Geometry: final body of the model. Coordinates: model frame, mm. A direction names the side the tool comes from. Give positions to 0.01 mm unless a question says otherwise; leave off trailing zeros. Order: outer loops, then holes, each group sorted by start corner. A loop starts at its lowest first (then second) coordinate and runs counter-clockwise, first axis right, second up. Notation, with made-up numbers: (-40, 50.25) - (-25, 50.25) arc R7 cw to (-25, 54.25) - close; hole circle Ø11 at (40, -31.5). An arc over 180 degrees is marked (long way). Put each result on its own line as item: value. Start each with the question number.
1. Section A-A on y = 11.5. Return the cut outline in (x, z).
2. Ray query, line 1 along X through (y, z) = (3, 10.75); line 2 along Y through (x, z) = (27.5, 8.25); line 3 along Y through (x, z) = (-3.5, 4.5). Return the intervals inside material, ascending. Write a range as from..to.
3. Mould query, pull axis X, two halves, no side actions, for faces 1 (the flat face through (-31, 12.55, 6)), 2 (the flat face through (26, -1.25, 6)), 3 (the flat face through (-34.25, 7, 6)), 4 (the cylindrical face through (-29.626, 12.906, 6.084)). Classes: pulls with the +X half, pulls with the -X half, needs draft (parallel to the pull), parting line crosses it, or undercut.
4. Section C-C on x = 14. Return the cut outline in (y, z), plus the area to 3 significant figures.
5. First-contact query: P1, Ø3.5, axis at x = -26, z = 5.5, coming from the -Y side; P2, Ø2, axis at x = 23, z = 3.5, coming from the -Y side; P3, Ø1.9, axis at y = -3.5, z = 7, coming from the -X side. Flat tips, straight axial feed; report the tip coordinate or a pass-through.
6. Section D-D on y = -4.5. Return the cut outline in (x, z), plus the area to 3 significant figures.
7. Set-up query: faces 5 (the cylindrical face through (-29.606, 14.674, 6.084)), 6 (the flat face through (31.75, 7, 6)), 7 (the flat face through (-6.25, -4, 6)). Return all of +Z, -Z, +X, -X, +Y, -Y with unobstructed straight access to the full face (end or side cutting, diameter ignored); none if empty.
from build123d import *

# Parameters (mm, degrees)
F0_W     = 22
F0_H     = 5
F1_DEPTH = 12
F2_W     = 12.5
F2_H     = 3.8
F3_DEPTH = 12
F4_R     = 5
F5_R     = 1.24999


# Not quite as in the source:
# - a fillet or chamfer is up to 0.001 mm smaller than in the source, because OpenCascade refuses the exact size


with BuildPart() as f1:
    # F0 (on Top) → F1 (new body)
    with BuildSketch(Plane.XY):
        Polygon((31.75, -1.25), (31.75, 1.25), (-31.75, 1.25), (-31.75, -1.25), (-16, -1.25), (-11, -1.25), (11, -1.25), (16, -1.25), align=None)
        Polygon((31.75, 12.55), (31.75, 1.25), (31.75, -1.25), (34.25, -1.25), (34.25, 12.55), align=None)
        Polygon((-31.75, -1.25), (-31.75, 1.25), (-31.75, 12.55), (-34.25, 12.55), (-34.25, -1.25), align=None)
        Polygon((29.25, 12.55), (31.75, 12.55), (34.25, 12.55), (34.25, 15.05), (29.25, 15.05), align=None)
        Polygon((-34.25, 12.55), (-31.75, 12.55), (-29.25, 12.55), (-29.25, 15.05), (-34.25, 15.05), align=None)
        with BuildLine():
            ThreePointArc((11, -6.25), (14.5355339059, -4.7855339059), (16, -1.25))
            Line((16, -1.25), (11, -1.25))
            Line((11, -1.25), (11, -6.25))
        make_face()
        with BuildLine():
            Line((-11, -1.25), (-16, -1.25))
            ThreePointArc((-16, -1.25), (-14.5355339059, -4.7855339059), (-11, -6.25))
            Line((-11, -6.25), (-11, -1.25))
        make_face()
        with Locations((0, -3.75)):
            Rectangle(F0_W, F0_H)
    extrude(amount=F1_DEPTH)

    # F2 (on face) → F3 (cut, through all)
    with BuildSketch(Plane.XY.offset(12)):
        with Locations((0, -4.35)):
            Rectangle(F2_W, F2_H)
    extrude(amount=-F3_DEPTH, mode=Mode.SUBTRACT)

    # F4
    f4_edges = [f1.edges().sort_by_distance(p)[0] for p in [
        (16, -1.25, 6),
        (-16, -1.25, 6),
    ]]
    fillet(f4_edges, radius=F4_R)

    # F5 (radius 1.25 in the source; OpenCascade refuses exactly that, so slightly less here)
    f5_edges = [f1.edges().sort_by_distance(p)[0] for p in [
        (-34.25, -1.25, 6),
        (34.25, -1.25, 6),
        (-34.25, 15.05, 6),
        (-29.25, 15.05, 6),
        (-29.25, 12.55, 6),
        (29.25, 12.55, 6),
        (29.25, 15.05, 6),
        (34.25, 15.05, 6),
    ]]
    fillet(f5_edges, radius=F5_R)


solid = f1.part
Resolved:
1. outline: (-34.25, 0) - (-31.75, 0) - (-31.75, 12) - (-34.25, 12) - close; (31.75, 0) - (34.25, 0) - (34.25, 12) - (31.75, 12) - close
2. line 1: -34.25..-31.75, 31.75..34.25
2. line 2: -1.25..1.25
2. line 3: -2.45..1.25
3. face 1: undercut
3. face 2: needs draft
3. face 3: pulls with the -X half
3. face 4: undercut
4. outline: (-5.25, 0) - (1.25, 0) - (1.25, 12) - (-5.25, 12) - close
4. area: 78.0 mm^2
5. P1: y = -1.25
5. P2: y = -1.25
5. P3: x = -16.3
6. outline: (-14.8, 0) - (-6.25, 0) - (-6.25, 12) - (-14.8, 12) - close; (6.25, 0) - (14.8, 0) - (14.8, 12) - (6.25, 12) - close
6. area: 205 mm^2
7. face 5: +Z, -Z, +Y
7. face 6: +Z, -Z
7. face 7: +Z, -Z, -Y
